Can you work these out from the model? Positions are in its coordinate system, mm. Face numbers are marked on the shaded views. Round coordinates to 2 decimals unless told otherwise and drop trailing zeros. Order: outer loops, then holes, each group sorted by start corner. A loop starts at its lowest first (then second) coordinate and runs counter-clockwise, first axis right, second up. Notation, with made-up numbers: M 37,73.5 L 50,73.5 A20 ccw 50,108.5 Z; hole C -40,87.25 d11. An arc over 180 degrees is marked long. One line per question, with ' | ' between items.
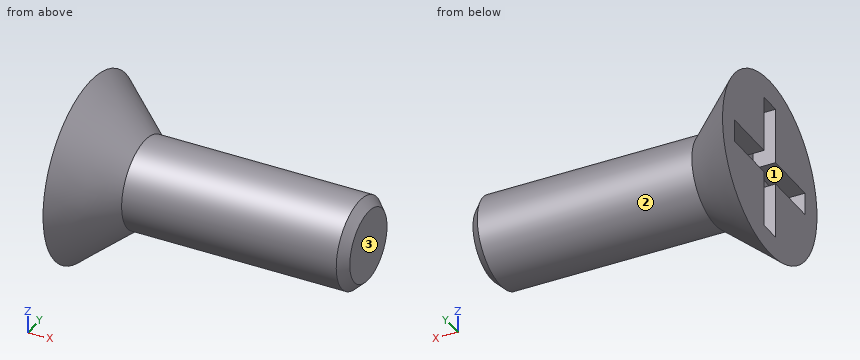
```python
from build123d import *

# Parameters (mm, degrees)
SKETCH2_W          = 2
SKETCH2_H          = 2
SKETCH2_H_2        = 5
SKETCH2_W_2        = 5
CUT_EXTRUDE1_DEPTH = 2


with BuildPart() as part:
    # Sketch1 → Revolve1 (revolve)
    with BuildSketch(Plane.XY, mode=Mode.PRIVATE) as revolve1_sk:
        Polygon((522.668754, 269.497429), (523.461488, 268.705203), (523.461488, 265.527536), (498.7671, 265.527536), (498.7671, 273.592163), (503.618754, 269.497429), align=None)
    revolve(revolve1_sk.sketch.rotate(Axis((523.461488, 265.527536, 0), (-1, 0, 0)), 90), axis=Axis((523.461488, 265.527536, 0), (-1, 0, 0)))

    # Sketch2 → Cut-Extrude1 (cut)
    with BuildSketch(Plane.ZY.offset(-498.7671)):
        with Locations((0, 265.527536)):
            Rectangle(SKETCH2_W, SKETCH2_H)
        with Locations((0, 269.027536)):
            Rectangle(SKETCH2_W, SKETCH2_H_2)
        with Locations((-3.5, 265.527536)):
            Rectangle(SKETCH2_W_2, SKETCH2_H)
        with Locations((3.5, 265.527536)):
            Rectangle(SKETCH2_W_2, SKETCH2_H)
        with Locations((0, 262.027536)):
            Rectangle(SKETCH2_W, SKETCH2_H_2)
    extrude(amount=-CUT_EXTRUDE1_DEPTH, mode=Mode.SUBTRACT)


solid = part.part
```
(1) Will these pins go through, and if not, where does the flat tip stop? pin 1 Ø2 at (x, z) = (499.5, 3.5) entering from -Y; pin 2 Ø0.6 at (x, y) = (500, 269) entering from +Z; pin 3 Ø1 at (x, y) = (499.5, 269) entering from -Z; pin 4 Ø1.6 at (x, z) = (499.5, 0) entering from -Y.
Final values:
pin 1: y = 257.97 | pin 2: z = 6.44 | pin 3: z = -7.12 | pin 4: y = 257.46
(2) Please list where these lines run through material, in increasing order: probe 1 along Y at (x, z) = (510.25, 0); probe 2 along X at (y, z) = (268.25, 0.75); probe 3 along Y at (x, z) = (510.25, -1.5). Write a range as [from, to].
Final values:
probe 1: [261.56, 269.5] | probe 2: [500.77, 523.46] | probe 3: [261.85, 269.2]
(3) If we section it at A-A on z = 0: Please give me the cut outline in (x, y), plus the area to 3 significant figures.
Final values:
outline: M 498.77,257.46 L 503.62,261.56 L 522.67,261.56 L 523.46,262.35 L 523.46,268.71 L 522.67,269.5 L 503.62,269.5 L 498.77,273.59 L 498.77,271.53 L 500.77,271.53 L 500.77,259.53 L 498.77,259.53 Z | area: 191 mm^2
(4) If we section it at B-B on x = 518: Please give me the cut outline in (y, z), plus the area to 3 significant figures.
Final values:
outline: C 265.53,0 d7.94 | area: 49.5 mm^2
(5) Thinking about a two-plate mould opening in Y: for the marked faces 1, 2 and 3, which applies, released by +Y, released by -Y, zero draft, split by the parting line, or undercut?
Final values:
face 1: undercut | face 2: split by the parting line | face 3: zero draft
